Job drawing, mm, ordinate dimensions from the low corner. One solid piece. Coordinates: 2 decimals unless noted, no trailing zeros. Write each loop counter-clockwise with the first axis right and the second up, starting at its lowest first coordinate (ties: lowest second). Pieces come first, ordered by that corner, then holes. Notation, with made-up numbers: (-31.5, 31.5) - (15.5, 31.5) arc R13 cw to (15.5, 45.5) - close; hole circle Ø9 at (1, -31.75). An arc over 180 degrees is marked (long way). Use a Markdown table: item, result.
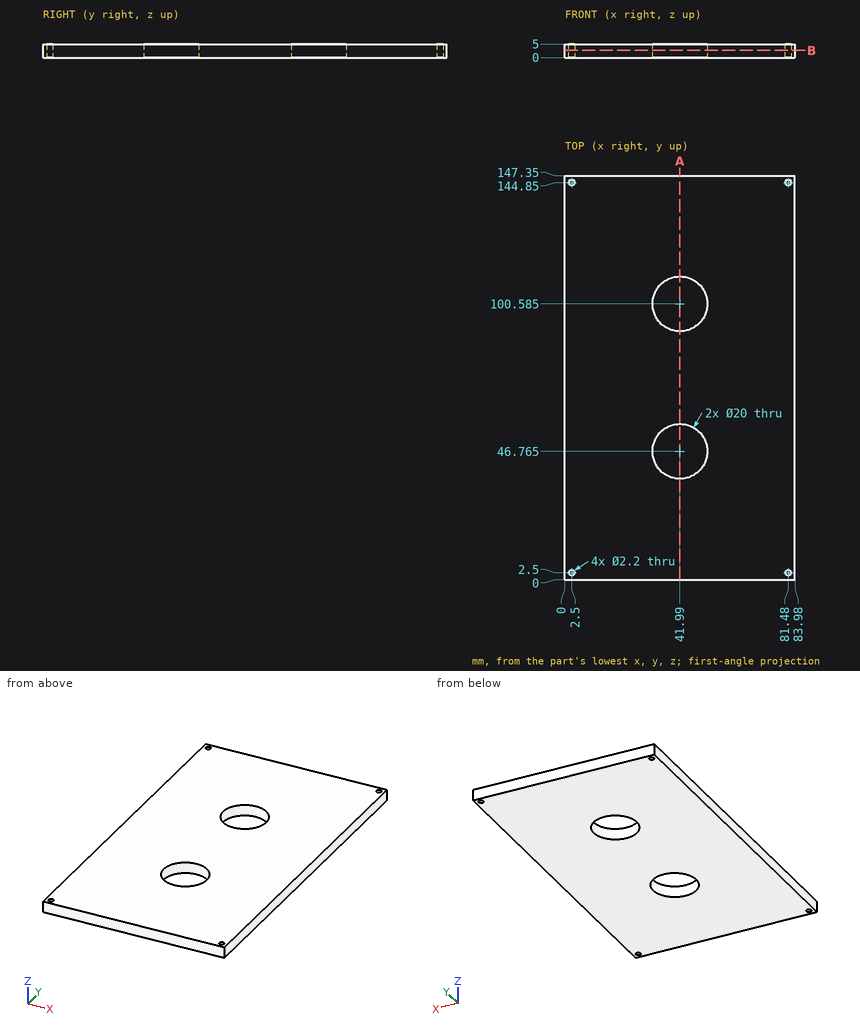
Item 1: Band-saw the part on B-B, the plane z = 2.7. Give the cut face in (x, y) (3 decimals).
From the geometry:
| item | result |
|---|---|
| outline | (0, 0) - (83.98, 0) - (83.98, 147.35) - (0, 147.35) - close; hole circle Ø2.2 at (2.5, 2.5); hole circle Ø2.2 at (2.5, 144.85); hole circle Ø20 at (41.99, 46.765); hole circle Ø20 at (41.99, 100.585); hole circle Ø2.2 at (81.48, 2.5); hole circle Ø2.2 at (81.48, 144.85) |
Item 2: Drill centre lines: probe 1 along Y at (x, z) = (81.48, 1.3); probe 2 along Y at (x, z) = (41.99, 1.4) (3 decimals). Where is each one in solid material? Low to high.
From the geometry:
| item | result |
|---|---|
| probe 1 | 0 to 1.4, 3.6 to 143.75, 145.95 to 147.35 |
| probe 2 | 0 to 36.765, 56.765 to 90.585, 110.585 to 147.35 |
Item 3: Drop a flat-ended pin along its axis: P1, Ø18, axis at x = 41.99, y = 46.765, coming from the -Z side. Give the stop position or say it passes through.
From the geometry:
| item | result |
|---|---|
| P1 | through |
Item 4: Band-saw the part on A-A, the plane x = 41.99. Give the cut face in (y, z) (3 decimals).
From the geometry:
| item | result |
|---|---|
| outline | (0, 0) - (36.765, 0) - (36.765, 5) - (0, 5) - close; (56.765, 0) - (90.585, 0) - (90.585, 5) - (56.765, 5) - close; (110.585, 0) - (147.35, 0) - (147.35, 5) - (110.585, 5) - close |
